from build123d import *

# Parameters (mm, degrees)
SKETCH1_R         = 34
BODY_DEPTH        = 74
SKETCH2_R         = 32.1
SLEEVE_BORE_DEPTH = 30
SKETCH3_R         = 30
CHAMBER_DEPTH     = 40
BASE_CORNER_R     = 2


with BuildPart() as part:
    # Sketch1 → Body (new body)
    with BuildSketch(Plane.XY):
        Circle(SKETCH1_R)
    extrude(amount=BODY_DEPTH)

    # Sketch2 → Sleeve_bore (cut)
    with BuildSketch(Plane.XY.offset(44)):
        Circle(SKETCH2_R)
    extrude(amount=SLEEVE_BORE_DEPTH, mode=Mode.SUBTRACT)

    # Sketch3 → Chamber (cut)
    with BuildSketch(Plane.XY.offset(4)):
        Circle(SKETCH3_R)
    extrude(amount=CHAMBER_DEPTH, mode=Mode.SUBTRACT)

    # Base_corner
    base_corner_edges = [part.edges().sort_by_distance(p)[0] for p in [
        (-30, 0, 4),
    ]]
    fillet(base_corner_edges, radius=BASE_CORNER_R)


solid = part.part
Geometry check sheet. Reference: the model listing, model coordinates, mm. A direction names the side the tool comes from. Coordinates: 2 decimals unless noted, no trailing zeros. Order: outer loops, then holes, each group sorted by start corner. A loop starts at its lowest first (then second) coordinate and runs counter-clockwise, first axis right, second up. Notation, with made-up numbers: M 70,-23 L 110,-23 A29 cw 110,12 Z; hole C 50,32.5 d3. An arc over 180 degrees is marked long. Use CSV: the item, a comma, the result in double quotes.
Item 1: Mould release check, pull along X, two halves, no side actions. Record for faces 1 (the flat face through (19, -24, 44)), 2 (the flat face through (0, 0, 0)), 3 (the cylindrical face through (18.28, 28.67, 36.48)): pulls with the +X half, pulls with the -X half, needs draft (parallel to the pull), parting line crosses it, or undercut.
Returned:
face 1,"undercut"
face 2,"needs draft"
face 3,"parting line crosses it"
Item 2: Thickness scan on line 1 along Y through (x, z) = (0, 54); line 2 along Y through (x, z) = (0, 31); line 3 along Z through (x, y) = (21, -8). Record the ranges inside material, lowest first.
Returned:
line 1,"y = -34 to -32.1, 32.1 to 34"
line 2,"y = -34 to -30, 30 to 34"
line 3,"z = 0 to 4"
Item 3: Cross-section at A-A on z = 11. Record the cut outline in (x, y).
Returned:
outline,"C 0,0 d68; hole C 0,0 d60"
Item 4: Gauge pin test, flat ends, axial feed: pin 1 Ø12 at (x, z) = (25.5, 53) entering from +Y; pin 2 Ø1 at (x, z) = (-5.5, 57) entering from -Y; pin 3 Ø4 at (x, y) = (-1.5, 0.5) entering from +Z. Record the tip position at first contact, or that the pin passes through.
Returned:
pin 1,"stops at y = 27.85"
pin 2,"stops at y = -33.63"
pin 3,"stops at z = 4"
Item 5: Cross-section at B-B on x = 0. Record the cut outline in (y, z), then the cut area to 3 significant figures.
Returned:
outline,"M -34,0 L 34,0 L 34,74 L 32.1,74 L 32.1,44 L 30,44 L 30,6 A2 cw 28,4 L -28,4 A2 cw -30,6 L -30,44 L -32.1,44 L -32.1,74 L -34,74 Z"
area,"708 mm2"
Item 6: Tool access check on faces 4 (the flat face through (30, -12, 74)), 5 (the cylindrical face through (-29.97, 1.32, 24.73)). Record the directions out of +Z, -Z, +X, -X, +Y, -Y that give a thin tool (end or side, any length) a straight path to the whole face; none if there is none.
Returned:
face 4,"+Z, +X, -X, +Y, -Y"
face 5,"+Z"
